Geometry: final body of the model. Coordinates: model frame, mm. Face numbers are marked on the shaded views. A direction names the side the tool comes from. Round coordinates to 2 decimals unless told otherwise and drop trailing zeros. Loops run counter-clockwise (first coordinate to the right, second up) from the corner with the lowest first, then second, coordinate; pieces in that order, holes last. Notation, with made-up numbers: (6, 78) - (36, 78) arc R16 cw to (36, 100) - close; hole circle Ø1 at (2.25, 83). An arc over 180 degrees is marked (long way). Return JSON: item names as keys, results as strings. Group by question number.
1. First-contact query: pin 1 Ø3.5 at (x, z) = (-0.5, 2) entering from -Y; pin 2 Ø4 at (x, y) = (-1.5, 0) entering from -Z; pin 3 Ø4 at (x, y) = (1.5, -1) entering from +Z; pin 4 Ø8 at (x, z) = (2.5, -11.5) entering from +Y. Flat tips, straight axial feed; report the tip coordinate or a pass-through.
2. Material intervals for probe 1 along Z at (x, y) = (3.5, 1.25); probe 2 along Y at (x, z) = (-18, -55); probe 3 along Z at (x, y) = (-10.5, -0.75), sorted ascending.
3. Section A-A on x = -8.5. Return loops of the section in (y, z), and give its area (3 significant figures).
4. Section B-B on z = -1. Return loops of the section in (x, y).
5. Section D-D on z = -33. Return loops of the section in (x, y), and give its area (3 significant figures).
6. Section C-C on x = -17.78. Return loops of the section in (y, z), and give its area (3 significant figures).
7. Set-up query: the marked faces 1, 2 and 3. Return all of +Z, -Z, +X, -X, +Y, -Y with unobstructed straight access to the full face (end or side cutting, diameter ignored); none if empty.
from build123d import *

# Parameters (mm, degrees)
F0_W           = 12.7
F0_H           = 12.1539
F1_DEPTH       = 2.2606
F2_DEPTH       = 4.1275
F3_W           = 3.6068
F3_H           = 11.2395
F4_DEPTH       = 12.7
F5_DEPTH       = 12.7
F6_R           = 0.508
F7_W           = 1.7526
F7_H           = 11.1379
F8_DEPTH       = 12.446
F10_DEPTH      = 9.398
F10_DEPTH_BACK = 0.508
F11_R          = 2.3495
F12_DEPTH      = 44.45


with BuildPart() as f1:
    # F0 (on Front) → F1 (new body, symmetric)
    with BuildSketch(Plane.XZ):
        Rectangle(F0_W, F0_H)
    extrude(amount=F1_DEPTH, both=True)

    # F0 (on Front) → F2 (join, symmetric)
    with BuildSketch(Plane.XZ):
        Polygon((-6.35, -8.128), (-6.35, -6.07695), (-6.35, 6.07695), (-6.35, 8.128), (-21.59, 8.128), (-21.59, -8.128), align=None)
    extrude(amount=F2_DEPTH, both=True)

    # F3 (on face) → F4 (cut)
    with BuildSketch(Plane.YZ.offset(6.35)):
        Rectangle(F3_W, F3_H)
    extrude(amount=-F4_DEPTH, mode=Mode.SUBTRACT)

    # F3 (on face) → F5 (cut)
    with BuildSketch(Plane.YZ.offset(6.35)):
        Rectangle(F3_W, F3_H)
    extrude(amount=-F5_DEPTH, mode=Mode.SUBTRACT)

    # F6
    f6_edges = [f1.edges().sort_by_distance(p)[0] for p in [
        (-6.35, -4.1275, 0),
        (-13.97, -4.1275, 8.128),
        (-21.59, -4.1275, 0),
        (-13.97, -4.1275, -8.128),
        (-6.35, 4.1275, 0),
        (-13.97, 4.1275, 8.128),
        (-21.59, 4.1275, 0),
        (-13.97, 4.1275, -8.128),
        (-21.59, 0, -8.128),
        (-21.59, 0, 8.128),
        (-6.35, 0, 8.128),
        (-6.35, 0, -8.128),
    ]]
    fillet(f6_edges, radius=F6_R)

    # F7 (on face) → F8 (join)
    with BuildSketch(Plane.YZ.offset(-6.35)):
        with Locations((-0.8763, 0)):
            Rectangle(F7_W, F7_H)
    extrude(amount=F8_DEPTH)

    # F9 (on face) → F10 (join, two sides)
    with BuildSketch(Plane(origin=(0, 0, -8.128), x_dir=(1, 0, 0), z_dir=(0, 0, -1))) as f10_sk:
        with BuildLine():
            ThreePointArc((-13.97, 0), (-17.78, 3.81), (-21.59, 0))
            Line((-21.59, 0), (-13.97, 0))
        make_face()
        with BuildLine():
            Line((-13.97, 0), (-21.59, 0))
            ThreePointArc((-21.59, 0), (-17.78, -3.81), (-13.97, 0))
        make_face()
    extrude(amount=F10_DEPTH)
    extrude(f10_sk.sketch, amount=-F10_DEPTH_BACK)

    # F11 (on face) → F12 (join)
    with BuildSketch(Plane(origin=(0, 0, -17.526), x_dir=(1, 0, 0), z_dir=(0, 0, -1))):
        with Locations((-17.78, 0)):
            Circle(F11_R)
    extrude(amount=F12_DEPTH)


solid = f1.part
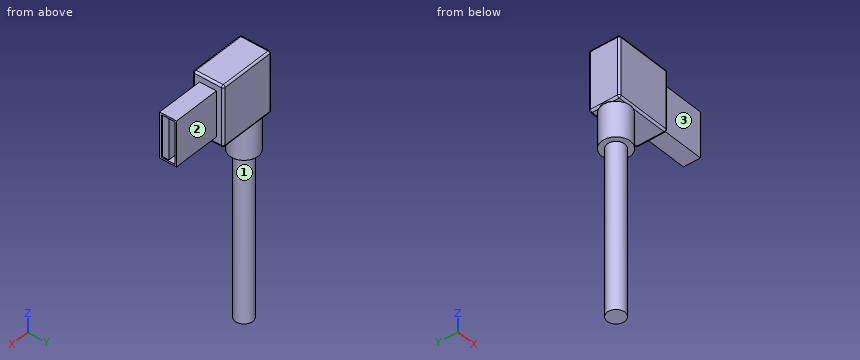
Taken from the geometry:
{
 "1": {"pin 1": "y = -2.26", "pin 2": "z = -6.08", "pin 3": "z = 6.08", "pin 4": "through"},
 "2": {"probe 1": "-6.08 to -5.62, 5.62 to 6.08", "probe 2": "-2.34 to 2.34", "probe 3": "-8.13 to 8.13"},
 "3": {"outline": "(-4.13, -7.62) arc R0.51 ccw to (-3.62, -8.13) - (3.62, -8.13) arc R0.51 ccw to (4.13, -7.62) - (4.13, 7.62) arc R0.51 ccw to (3.62, 8.13) - (-3.62, 8.13) arc R0.51 ccw to (-4.13, 7.62) - close", "area": "134 mm2"},
 "4": {"outline": "(-21.59, -3.62) arc R0.51 ccw to (-21.08, -4.13) - (-6.86, -4.13) arc R0.51 ccw to (-6.35, -3.62) - (-6.35, -2.26) - (6.35, -2.26) - (6.35, -1.8) - (-6.35, -1.8) - (-6.35, -1.75) - (6.1, -1.75) - (6.1, 0) - (-6.35, 0) - (-6.35, 1.8) - (6.35, 1.8) - (6.35, 2.26) - (-6.35, 2.26) - (-6.35, 3.62) arc R0.51 ccw to (-6.86, 4.13) - (-21.08, 4.13) arc R0.51 ccw to (-21.59, 3.62) - close"},
 "5": {"outline": "circle Ø4.7 at (-17.78, 0)", "area": "17.3 mm2"},
 "6": {"outline": "(-4.13, -7.62) arc R0.51 ccw to (-3.81, -8.09) - (-3.81, -17.53) - (-2.35, -17.53) - (-2.35, -61.98) - (2.35, -61.98) - (2.35, -17.53) - (3.81, -17.53) - (3.81, -8.09) arc R0.51 ccw to (4.13, -7.62) - (4.13, 7.62) arc R0.51 ccw to (3.62, 8.13) - (-3.62, 8.13) arc R0.51 ccw to (-4.13, 7.62) - close", "area": "414 mm2"},
 "7": {"face 1": "-Z", "face 2": "+Z, -Z, +X, +Y", "face 3": "+Z, -Z, +X, -Y"}
}
